```python
from build123d import *

# Parameters (mm, degrees)
SKETCH1_W                    = 15.6
SKETCH1_H                    = 16
BOSS_EXTRUDE1_DEPTH          = 6.95
SKETCH1_3_W                  = 4.4
SKETCH1_3_H                  = 16
BOSS_EXTRUDE2_DEPTH          = 16.95
BOSS_EXTRUDE3_START          = 16.95
SKETCH1_4_W                  = 15.6
SKETCH1_4_H                  = 16
BOSS_EXTRUDE3_DEPTH          = 6.95
SKETCH2_R                    = 2.6
CUT_EXTRUDE1_DEPTH           = 3.9
CUT_EXTRUDE1_DRAFT           = -1.5
CUT_EXTRUDE1_PROFILE_2_DEPTH = 3.9
CUT_EXTRUDE1_PROFILE_2_DRAFT = -1.5
SKETCH2_3_R                  = 1.6
CUT_EXTRUDE2_DEPTH           = 84.804594146
SKETCH3_R                    = 1
CUT_EXTRUDE3_DEPTH           = 79.499442673
SKETCH3_3_R                  = 2.1
CUT_EXTRUDE4_DEPTH           = 2
CUT_EXTRUDE5_START           = -23.9
SKETCH2_4_R                  = 2.6
CUT_EXTRUDE5_DEPTH           = 3.9
CUT_EXTRUDE5_DRAFT           = 1.5
CUT_EXTRUDE5_PROFILE_2_DEPTH = 3.9
CUT_EXTRUDE5_PROFILE_2_DRAFT = 1.5


with BuildPart() as part:
    # Sketch1 → Boss-Extrude1 (new body)
    with BuildSketch(Plane(origin=(-11.95, 0, 0), x_dir=(0, 0, -1), z_dir=(1, 0, 0))):
        with Locations((18.2, 68)):
            Rectangle(SKETCH1_W, SKETCH1_H)
    extrude(amount=BOSS_EXTRUDE1_DEPTH)

    # Sketch1<3> → Boss-Extrude2 (add)
    with BuildSketch(Plane(origin=(-11.95, 0, 0), x_dir=(0, 0, -1), z_dir=(1, 0, 0))):
        with Locations((23.8, 68)):
            Rectangle(SKETCH1_3_W, SKETCH1_3_H)
    extrude(amount=BOSS_EXTRUDE2_DEPTH)

    # Sketch1<4> → Boss-Extrude3 (add)
    with BuildSketch(Plane(origin=(-11.95, 0, 0), x_dir=(0, 0, -1), z_dir=(1, 0, 0)).offset(BOSS_EXTRUDE3_START)):
        with Locations((18.2, 68)):
            Rectangle(SKETCH1_4_W, SKETCH1_4_H)
    extrude(amount=BOSS_EXTRUDE3_DEPTH)


with BuildPart() as cut_extrude1_tool:
    # Sketch2 → Cut-Extrude1 (with draft: the straight prism first)
    with BuildSketch(Plane.ZY.offset(11.95)):
        with Locations((-21.811399183, 64.296000838)):
            Circle(SKETCH2_R)
    extrude(amount=-CUT_EXTRUDE1_DEPTH)
    # Cut-Extrude1: the draft: its side faces are tilted about the plane it starts from
    cut_extrude1_sides = [cut_extrude1_tool.faces().sort_by_distance(p)[0] for p in [
        (-10, 64.296000838, -24.411399183),
    ]]
    draft(cut_extrude1_sides, Plane.ZY.offset(11.95), CUT_EXTRUDE1_DRAFT)


with BuildPart() as part_1:
    add(part.part)

    # Cut-Extrude1: cut by cut_extrude1_tool
    add(cut_extrude1_tool.part, mode=Mode.SUBTRACT)


with BuildPart() as cut_extrude1_profile_2_tool:
    # Sketch2 → Cut-Extrude1 profile 2 (with draft: the straight prism first)
    with BuildSketch(Plane.ZY.offset(11.95)):
        with Locations((-14.588600817, 71.703999162)):
            Circle(SKETCH2_R)
    extrude(amount=-CUT_EXTRUDE1_PROFILE_2_DEPTH)
    # Cut-Extrude1 profile 2: the draft: its side faces are tilted about the plane it starts from
    cut_extrude1_profile_2_sides = [cut_extrude1_profile_2_tool.faces().sort_by_distance(p)[0] for p in [
        (-10, 71.703999162, -17.188600817),
    ]]
    draft(cut_extrude1_profile_2_sides, Plane.ZY.offset(11.95), CUT_EXTRUDE1_PROFILE_2_DRAFT)


with BuildPart() as part_2:
    add(part_1.part)

    # Cut-Extrude1 profile 2: cut by cut_extrude1_profile_2_tool
    add(cut_extrude1_profile_2_tool.part, mode=Mode.SUBTRACT)

    # Sketch2<3> → Cut-Extrude2 (cut, through all)
    with BuildSketch(Plane.ZY.offset(11.95)):
        with Locations(Location((-21.811399183, 64.296000838, 0), (0, 0, 270))):
            Circle(SKETCH2_3_R)
        with Locations(Location((-14.588600817, 71.703999162, 0), (0, 0, 270))):
            Circle(SKETCH2_3_R)
    extrude(amount=-CUT_EXTRUDE2_DEPTH, mode=Mode.SUBTRACT)

    # Sketch3 → Cut-Extrude3 (cut, through all)
    with BuildSketch(Plane(origin=(0, 0, -26), x_dir=(-1, 0, 0), z_dir=(0, 0, -1))):
        with Locations(Location((3, 73.05466329, 0), (0, 0, 90))):
            Circle(SKETCH3_R)
        with Locations(Location((-3, 63.05466329, 0), (0, 0, 90))):
            Circle(SKETCH3_R)
    extrude(amount=-CUT_EXTRUDE3_DEPTH, mode=Mode.SUBTRACT)

    # Sketch3<3> → Cut-Extrude4 (cut)
    with BuildSketch(Plane(origin=(0, 0, -26), x_dir=(-1, 0, 0), z_dir=(0, 0, -1))):
        with Locations(Location((3, 73.05466329, 0), (0, 0, 90))):
            Circle(SKETCH3_3_R)
        with Locations(Location((-3, 63.05466329, 0), (0, 0, 90))):
            Circle(SKETCH3_3_R)
    extrude(amount=-CUT_EXTRUDE4_DEPTH, mode=Mode.SUBTRACT)


with BuildPart() as cut_extrude5_tool:
    # Sketch2<4> → Cut-Extrude5 (with draft: the straight prism first)
    with BuildSketch(Plane.ZY.offset(11.95).offset(CUT_EXTRUDE5_START)):
        with Locations((-21.811399183, 64.296000838)):
            Circle(SKETCH2_4_R)
    extrude(amount=CUT_EXTRUDE5_DEPTH)
    # Cut-Extrude5: the draft: its side faces are tilted about the plane it starts from
    cut_extrude5_sides = [cut_extrude5_tool.faces().sort_by_distance(p)[0] for p in [
        (10, 64.296000838, -24.411399183),
    ]]
    draft(cut_extrude5_sides, Plane.ZY.offset(11.95).offset(CUT_EXTRUDE5_START), CUT_EXTRUDE5_DRAFT)


with BuildPart() as part_3:
    add(part_2.part)

    # Cut-Extrude5: cut by cut_extrude5_tool
    add(cut_extrude5_tool.part, mode=Mode.SUBTRACT)


with BuildPart() as cut_extrude5_profile_2_tool:
    # Sketch2<4> → Cut-Extrude5 profile 2 (with draft: the straight prism first)
    with BuildSketch(Plane.ZY.offset(11.95).offset(CUT_EXTRUDE5_START)):
        with Locations((-14.588600817, 71.703999162)):
            Circle(SKETCH2_4_R)
    extrude(amount=CUT_EXTRUDE5_PROFILE_2_DEPTH)
    # Cut-Extrude5 profile 2: the draft: its side faces are tilted about the plane it starts from
    cut_extrude5_profile_2_sides = [cut_extrude5_profile_2_tool.faces().sort_by_distance(p)[0] for p in [
        (10, 71.703999162, -17.188600817),
    ]]
    draft(cut_extrude5_profile_2_sides, Plane.ZY.offset(11.95).offset(CUT_EXTRUDE5_START), CUT_EXTRUDE5_PROFILE_2_DRAFT)


with BuildPart() as part_4:
    add(part_3.part)

    # Cut-Extrude5 profile 2: cut by cut_extrude5_profile_2_tool
    add(cut_extrude5_profile_2_tool.part, mode=Mode.SUBTRACT)


solid = part_4.part
```
The listing builds one solid part. Answer for the finished solid, in the listing's coordinates (mm). A direction names the side the tool comes from. Round coordinates to 2 decimals unless told otherwise and drop trailing zeros. Loops run counter-clockwise (first coordinate to the right, second up) from the corner with the lowest first, then second, coordinate; pieces in that order, holes last.
Q1. Which of the six approach directions +Z, -Z, +X, -X, +Y, -Y give full straight-line access (tool end or side, diameter ignored) to faces 1 (the face through (-10.027, 66.824, -22.143)), 2 (the face through (0, 71, -21.6)), 3 (the face through (-2.37, 75.06, -25.01))?
Q2. Section C-C, the plane y = 68.75 is taken. Determine the outline of the cut face in (x, z).
Q3. Section B-B, the plane x = -3 is taken. Determine the outline of the cut face in (y, z), then the cut area to 3 significant figures.
Q4. For a pull along X with two mould halves and no side action, classify faces 4 (the face through (10.027, 74.232, -14.921)), 5 (the face through (6.5, 73.3, -14.5)), 6 (the face through (0, 61, -21.6)) as released by +X, released by -X, zero draft, split by the parting line, or undercut.
Q5. Find the intervals of material crossed by line 1 (X direction, y = 63, z = -25); line 2 (X direction, y = 63.5, z = -12.75); line 3 (Z direction, x = 0, y = 73), in increasing order.
Q6. Given pin 1 Ø0.8 at (x, y) = (-1, 61) entering from +Z; pin 2 Ø1.5 at (y, z) = (63.5, -22.5) entering from +X; pin 3 Ø3.5 at (y, z) = (64.3, -21.81) entering from -X, each flat-ended and moving along its own axis, determine where each tip first touches the part or whether it passes through.
Q7. Section A-A, the plane z = -11.5 is taken. Determine the outline of the cut face in (x, y).
Q8. Section D-D, the plane x = 1.5 is taken. Determine the outline of the cut face in (y, z).
Completed:
1. face 1: -X
1. face 2: +Z, +Y, -Y
1. face 3: -Z
2. outline: (-11.95, -26) - (11.95, -26) - (11.95, -10.4) - (5, -10.4) - (5, -21.6) - (-5, -21.6) - (-5, -10.4) - (-11.95, -10.4) - close
3. outline: (60, -26) - (70.95, -26) - (70.95, -24) - (72.05, -24) - (72.05, -21.6) - (65.88, -21.6) arc R1.6 cw (long way) to (62.71, -21.6) - (60, -21.6) - close; (74.05, -24) - (75.15, -24) - (75.15, -26) - (76, -26) - (76, -21.6) - (74.05, -21.6) - close
3. area: 52.5 mm2
4. face 4: released by +X
4. face 5: zero draft
4. face 6: undercut
5. line 1: x = -11.95 to 0.9, 5.1 to 11.95
5. line 2: x = -11.95 to -5, 5 to 11.95
5. line 3: z = -26 to -21.6
6. pin 1: stops at z = -21.6
6. pin 2: stops at x = 8.05
6. pin 3: stops at x = -8.05
7. outline: (-11.95, 60) - (-5, 60) - (-5, 76) - (-11.95, 76) - close; (5, 60) - (11.95, 60) - (11.95, 76) - (5, 76) - close
8. outline: (60, -26) - (61.58, -26) - (61.58, -24) - (64.52, -24) - (64.52, -26) - (76, -26) - (76, -21.6) - (65.88, -21.6) arc R1.6 cw (long way) to (62.71, -21.6) - (60, -21.6) - close
